Study the drawing (mm; zero at the part's minimum x, y, z) and answer. A direction names the side the tool comes from. Give positions to 0.01 mm unless a question says otherwise; leave off trailing zeros. Write each loop counter-clockwise with the first axis right and the second up, starting at its lowest first coordinate (ties: lowest second). Pieces come first, ordered by that corner, then holes. Notation, with made-up numbers: (-28.5, 79) - (-6.5, 79) arc R27 ccw to (-6.5, 113) - close; hole circle Ø2 at (7.25, 71). An arc over 180 degrees is marked (long way). Write each question's results on one line, items separated by ' | '. Start each with the question number.
Q1. For a pull along Z with two mould halves and no side action, classify the marked faces 1, 2 and 3 as pulls with the +Z half, pulls with the -Z half, needs draft (parallel to the pull), parting line crosses it, or undercut.
Q2. Find the intervals of material crossed by probe 1 along Y at (x, z) = (3.5, 2.2); probe 2 along Y at (x, z) = (2.75, 4.2); probe 3 along Z at (x, y) = (1.5, 12.25), in increasing order.
Q3. Section C-C (z = 2.5) is taken. Determine the outline of the cut face in (x, y), plus the area to 3 significant figures.
Q4. Flat-ended cylindrical pins translate along their axes: pin 1 Ø0.8 at (x, z) = (1.5, 2.5) entering from -Y; pin 2 Ø1.1 at (x, z) = (1.5, 2.5) entering from +Y. Find the tip coordinate at first contact, or state that the pin passes through.
Q5. Section A-A (y = 11) is taken. Determine the outline of the cut face in (x, z).
Q6. Section D-D (y = 8) is taken. Determine the outline of the cut face in (x, z), plus the area to 3 significant figures.
Q7. For the marked faces 4, 5 and 6, determine the directions among +Z, -Z, +X, -X, +Y, -Y from which every point of the face is accessible in a straight line to the end or side of a thin tool.
Q8. Section B-B (x = 3.5) is taken. Determine the outline of the cut face in (y, z), plus the area to 3 significant figures.
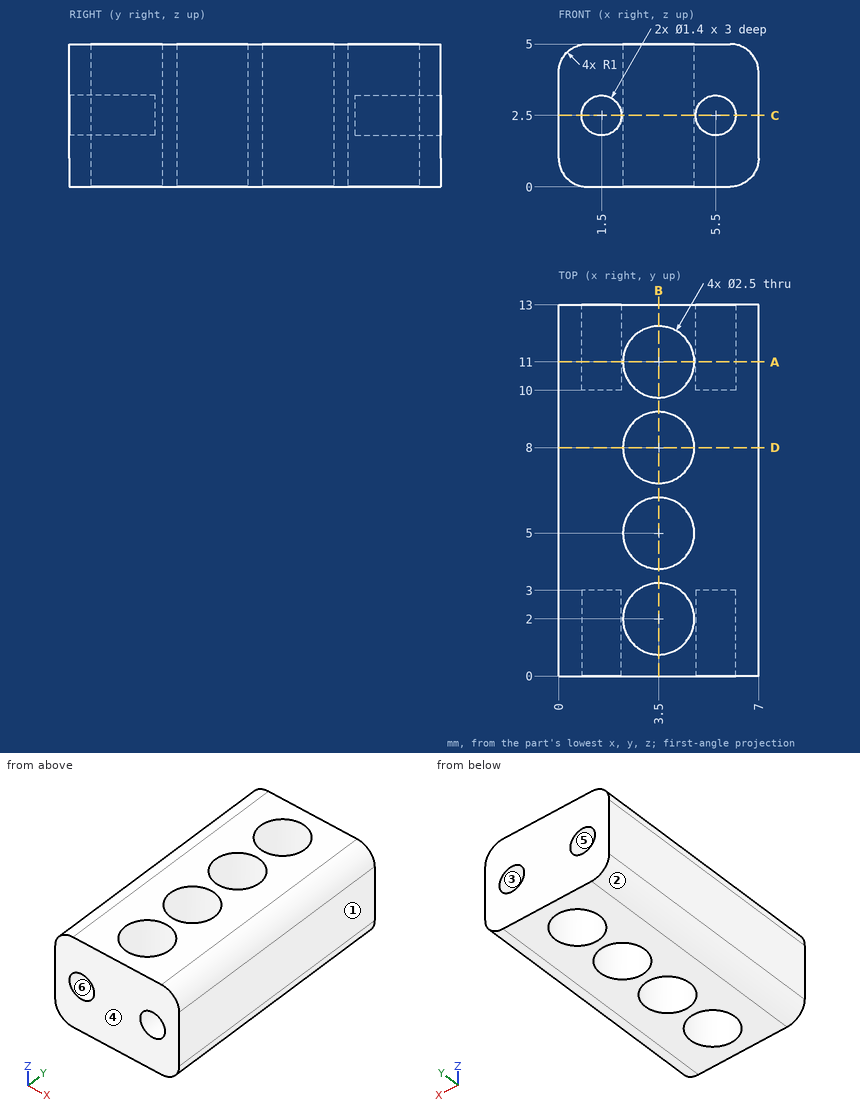
Answers below:
1) face 1: needs draft | face 2: pulls with the -Z half | face 3: undercut
2) probe 1: y = 0 to 0.75, 3.25 to 3.75, 6.25 to 6.75, 9.25 to 9.75, 12.25 to 13 | probe 2: y = 0 to 1, 3 to 4, 6 to 7, 9 to 10, 12 to 13 | probe 3: z = 0 to 1.8, 3.2 to 5
3) outline: (0, 0) - (0.8, 0) - (0.8, 3) - (2.2, 3) - (2.2, 0) - (4.8, 0) - (4.8, 3) - (6.2, 3) - (6.2, 0) - (7, 0) - (7, 13) - (6.2, 13) - (6.2, 10) - (4.8, 10) - (4.8, 13) - (2.2, 13) - (2.2, 10) - (0.8, 10) - (0.8, 13) - (0, 13) - close; hole circle Ø2.5 at (3.5, 2); hole circle Ø2.5 at (3.5, 5); hole circle Ø2.5 at (3.5, 8); hole circle Ø2.5 at (3.5, 11) | area: 54.6 mm2
4) pin 1: stops at y = 3 | pin 2: stops at y = 10
5) outline: (0, 1) arc R1 ccw to (1, 0) - (2.25, 0) - (2.25, 5) - (1, 5) arc R1 ccw to (0, 4) - close; (4.75, 0) - (6, 0) arc R1 ccw to (7, 1) - (7, 4) arc R1 ccw to (6, 5) - (4.75, 5) - close; hole circle Ø1.4 at (1.5, 2.5); hole circle Ø1.4 at (5.5, 2.5)
6) outline: (0, 1) arc R1 ccw to (1, 0) - (2.25, 0) - (2.25, 5) - (1, 5) arc R1 ccw to (0, 4) - close; (4.75, 0) - (6, 0) arc R1 ccw to (7, 1) - (7, 4) arc R1 ccw to (6, 5) - (4.75, 5) - close | area: 21.6 mm2
7) face 4: +Z, -Z, +X, -X, -Y | face 5: +Y | face 6: -Y
8) outline: (0, 0) - (0.75, 0) - (0.75, 5) - (0, 5) - close; (3.25, 0) - (3.75, 0) - (3.75, 5) - (3.25, 5) - close; (6.25, 0) - (6.75, 0) - (6.75, 5) - (6.25, 5) - close; (9.25, 0) - (9.75, 0) - (9.75, 5) - (9.25, 5) - close; (12.25, 0) - (13, 0) - (13, 5) - (12.25, 5) - close | area: 15.0 mm2
